The model under review builds one solid part; all positions refer to its coordinate system, in mm. A direction names the side the tool comes from. Round coordinates to 2 decimals unless told otherwise and drop trailing zeros. Order: outer loops, then holes, each group sorted by start corner. A loop starts at its lowest first (then second) coordinate and runs counter-clockwise, first axis right, second up.
```python
from build123d import *

# Parameters (mm, degrees)
F0_R     = 4.8
F1_DEPTH = 6.2
F2_R     = 4.8
F3_DEPTH = 5.5
F4_R     = 4.8
F5_DEPTH = 4
F6_R     = 5.1
F6_R_2   = 4.8
F7_DEPTH = 2.6
F8_R     = 2.15
F9_DEPTH = 18.301


with BuildPart() as f1:
    # F0 (on Top) → F1 (new body)
    with BuildSketch(Plane.XY):
        Circle(F0_R)
    extrude(amount=F1_DEPTH)

    # F2 (on face) → F3 (join)
    with BuildSketch(Plane.XY.offset(6.2)):
        Polygon((2.8867513459, -5), (5.7735026919, 0), (2.8867513459, 5), (-2.8867513459, 5), (-5.7735026919, 0), (-2.8867513459, -5), align=None)
        Circle(F2_R, mode=Mode.SUBTRACT)
        Circle(F2_R)
    extrude(amount=F3_DEPTH)

    # F4 (on face) → F5 (join)
    with BuildSketch(Plane.XY.offset(11.7)):
        Circle(F4_R)
    extrude(amount=F5_DEPTH)

    # F6 (on face) → F7 (join)
    with BuildSketch(Plane.XY.offset(15.7)):
        Circle(F6_R)
        Circle(F6_R_2, mode=Mode.SUBTRACT)
        Circle(F6_R_2)
    extrude(amount=F7_DEPTH)

    # F8 (on face) → F9 (cut, through all)
    with BuildSketch(Plane.XY.offset(18.3)):
        Circle(F8_R)
    extrude(amount=-F9_DEPTH, mode=Mode.SUBTRACT)


solid = f1.part
```
(1) Insertion check: pin 1 (1 mm diameter, centred on y = -1, z = 14, fed in from -X); pin 2 (4.5 mm diameter, centred on x = 0.5, z = 9.5, fed in from -Y); pin 3 (1.6 mm diameter, centred on x = -1, z = 10, fed in from +Y); pin 4 (3 mm diameter, centred on x = -0.5, y = 0, fed in from -Z). Each pin has a flat end and moves straight along its axis. Give the tip position at first contact, or say it passes through.
Data:
pin 1: stops at x = -4.77
pin 2: stops at y = -5
pin 3: stops at y = 5
pin 4: passes through
(2) Consider section A-A (x = 0). Write out the cut boundary in (y, z), and give its area (3 significant figures).
Data:
outline: (-5.1, 15.7) - (-4.8, 15.7) - (-4.8, 11.7) - (-5, 11.7) - (-5, 6.2) - (-4.8, 6.2) - (-4.8, 0) - (-2.15, 0) - (-2.15, 18.3) - (-5.1, 18.3) - close; (2.15, 0) - (4.8, 0) - (4.8, 6.2) - (5, 6.2) - (5, 11.7) - (4.8, 11.7) - (4.8, 15.7) - (5.1, 15.7) - (5.1, 18.3) - (2.15, 18.3) - close
area: 101 mm2
(3) To check wall thickness, follow probe 1 along Y at (x, z) = (0, 5.5); probe 2 along Z at (x, y) = (-2, -4.5); probe 3 along Y at (x, z) = (0, 10.25). State the ranges of each line that lie inside material, in increasing order.
Data:
probe 1: y = -4.8 to -2.15, 2.15 to 4.8
probe 2: z = 6.2 to 11.7, 15.7 to 18.3
probe 3: y = -5 to -2.15, 2.15 to 5
(4) Consider section D-D (x = -3.75). Write out the cut boundary in (y, z).
Data:
outline: (-3.5, 6.2) - (-3, 6.2) - (-3, 0) - (3, 0) - (3, 6.2) - (3.5, 6.2) - (3.5, 11.7) - (3, 11.7) - (3, 15.7) - (3.46, 15.7) - (3.46, 18.3) - (-3.46, 18.3) - (-3.46, 15.7) - (-3, 15.7) - (-3, 11.7) - (-3.5, 11.7) - close
(5) Consider section B-B (z = 8). Write out the cut boundary in (x, y).
Data:
outline: (-5.77, 0) - (-2.89, -5) - (2.89, -5) - (5.77, 0) - (2.89, 5) - (-2.89, 5) - close; hole circle Ø4.3 at (0, 0)
(6) For faces 5 (the flat face through (4.31, -2.535, 8.912)), 6 (the cylindrical face through (2.58, 4.05, 3.06)), 7 (the flat face through (-4.35, -2.465, 8.912)), 8 (the cylindrical face through (2.58, 4.05, 13.67)), list the 3-axis set-ups (+Z, -Z, +X, -X, +Y, -Y) from which the entire face can be reached by the end or side of a thin tool; tool diameter is ignored.
Data:
face 5: -Z, +X, -Y
face 6: -Z
face 7: -Z, -X, -Y
face 8: none
(7) Consider section C-C (y = 0.25). Write out the cut boundary in (x, z).
Data:
outline: (-5.63, 6.2) - (-4.79, 6.2) - (-4.79, 0) - (-2.14, 0) - (-2.14, 18.3) - (-5.09, 18.3) - (-5.09, 15.7) - (-4.79, 15.7) - (-4.79, 11.7) - (-5.63, 11.7) - close; (2.14, 0) - (4.79, 0) - (4.79, 6.2) - (5.63, 6.2) - (5.63, 11.7) - (4.79, 11.7) - (4.79, 15.7) - (5.09, 15.7) - (5.09, 18.3) - (2.14, 18.3) - close
(8) Draft analysis for pull direction Y (two halves, no side actions). For faces 1 (the cylindrical face through (-2.15, 0.09, 9.28)), 2 (the flat face through (0, -5, 9)), 3 (the flat face through (0, 5, 9)), 4 (the flat face through (5, 1, 11.7)), state which applies: pulls with the +Y half, pulls with the -Y half, needs draft (parallel to the pull), parting line crosses it, or undercut.
Data:
face 1: undercut
face 2: pulls with the -Y half
face 3: pulls with the +Y half
face 4: needs draft
